Design review of the part shown in the three views and the two pictorial views. Dimensions are in mm from the part's minimum x, y and z. A direction names the side the tool comes from. Coordinates: 2 decimals unless noted, no trailing zeros. Loops run counter-clockwise (first coordinate to the right, second up) from the corner with the lowest first, then second, coordinate; pieces in that order, holes last. Notation, with made-up numbers: (34.25, 61.5) - (47.25, 61.5) arc R20 cw to (47.25, 93.5) - close; hole circle Ø4 at (57.5, 72). An arc over 180 degrees is marked (long way). One line per question, with ' | ' between items.
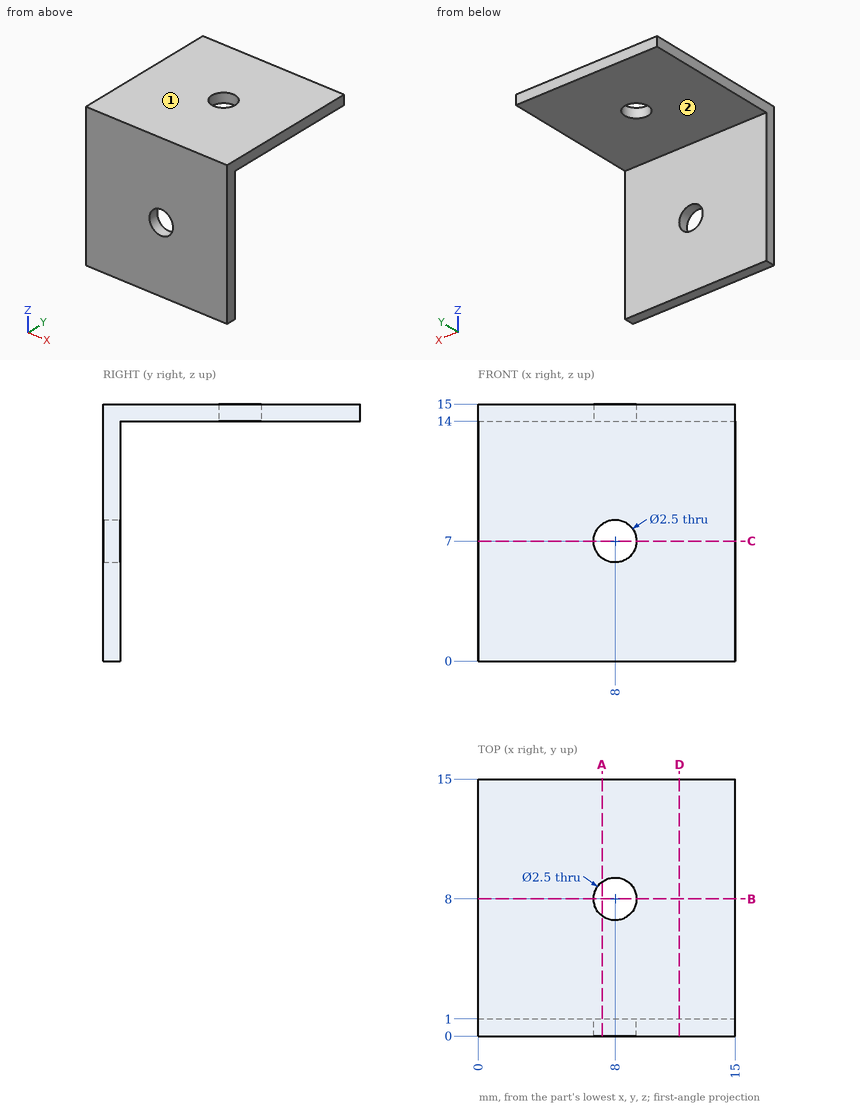
Q1. Tool access review of the marked faces 1 and 2: name each direction out of +Z, -Z, +X, -X, +Y, -Y from which nothing blocks a thin tool from reaching the whole face with its end or side.
Returned:
face 1: +Z, +X, -X, +Y, -Y | face 2: -Z, +X, -X, +Y
Q2. Take a section at B-B (y = 8). Give the boundary of the cut face in (x, z).
Returned:
outline: (0, 14) - (6.75, 14) - (6.75, 15) - (0, 15) - close; (9.25, 14) - (15, 14) - (15, 15) - (9.25, 15) - close
Q3. Take a section at D-D (x = 11.75). Give the boundary of the cut face in (y, z).
Returned:
outline: (0, 0) - (1, 0) - (1, 14) - (15, 14) - (15, 15) - (0, 15) - close
Q4. To check wall thickness, follow line 1 along X through (y, z) = (0.5, 7); line 2 along Z through (x, y) = (8, 0.2). State the ranges of each line that lie inside material, in increasing order.
Returned:
line 1: x = 0 to 6.75, 9.25 to 15 | line 2: z = 0 to 5.75, 8.25 to 15
Q5. Take a section at A-A (x = 7.25). Give the boundary of the cut face in (y, z).
Returned:
outline: (0, 0) - (1, 0) - (1, 6) - (0, 6) - close; (0, 8) - (1, 8) - (1, 14) - (7, 14) - (7, 15) - (0, 15) - close; (9, 14) - (15, 14) - (15, 15) - (9, 15) - close
Q6. Take a section at C-C (z = 7). Give the boundary of the cut face in (x, y), plus the area to 3 significant figures.
Returned:
outline: (0, 0) - (6.75, 0) - (6.75, 1) - (0, 1) - close; (9.25, 0) - (15, 0) - (15, 1) - (9.25, 1) - close | area: 12.5 mm²
Q7. For pin 1 (4 mm diameter, centred on x = 8, y = 8, fed in from -Z); pin 2 (1 mm diameter, centred on x = 11.5, z = 8, fed in from -Y), all flat-tipped, find the tip position at first contact; note any pin that passes through.
Returned:
pin 1: stops at z = 14 | pin 2: stops at y = 0
